Autodesk Inventor part; units mm, degrees
ref_plane "YZ Plane" through (0, 0, 0) normal (1, 0, 0) x (0, 1, 0)
ref_plane "XZ Plane" through (0, 0, 0) normal (0, 1, 0) x (-1, 0, 0)
ref_plane "XY Plane" through (0, 0, 0) normal (0, 0, 1) x (1, 0, 0)
sketch "Sketch1" plane through (0, 0, 0) normal (0, 1, 0) x (-1, 0, 0)
  line L0 (-600, 400) -> (600, 400)
  line L1 (600, 400) -> (600, -400)
  line L2 (600, -400) -> (-600, -400)
  line L3 (-600, -400) -> (-600, 400)
  line L4 (-600, 400) -> (600, -400) construction
  line L5 (600, 400) -> (-600, -400) construction
  point P0 (0, 0)
  dimension "d0" = 1200
  dimension "d1" = 800
extrude "Extrusion1" add sketch "Sketch1" along normal blind 35
sketch "Sketch2" plane through (0, 35, 0) normal (0, 1, 0) x (1, 0, 0)
  line L0 (-300, -215) -> (300, -215)
  line L1 (300, -215) -> (300, 215)
  line L2 (300, 215) -> (-300, 215)
  line L3 (-300, 215) -> (-300, -215)
  line L4 (-300, -215) -> (300, 215) construction
  line L5 (300, -215) -> (-300, 215) construction
  point P0 (0, 0)
  dimension "d8" = 430
  dimension "d9" = 600
extrude "Extrusion2" cut sketch "Sketch2" against normal blind 35
fillet "Fillet2" radius 10 4 edges at (0, 35, 400) (-600, 35, 0) (0, 35, -400) (600, 35, 0)
fillet "Fillet3" radius 10 8 edges at (597.0711, 32.0711, 397.0711) (600, 12.5, 400) (597.0711, 32.0711, -397.0711) (600, 12.5, -400) (-597.0711, 32.0711, 397.0711) (-600, 12.5, 400) (-597.0711, 32.0711, -397.0711) (-600, 12.5, -400)
properties part number "señales_tapa_x10"
Geometry check sheet. Reference: the model listing, model coordinates, mm. A direction names the side the tool comes from. Round coordinates to 2 decimals unless told otherwise and drop trailing zeros. Order: outer loops, then holes, each group sorted by start corner. A loop starts at its lowest first (then second) coordinate and runs counter-clockwise, first axis right, second up. Notation, with made-up numbers: (-32, -24.5) - (18, -24.5) arc R21 cw to (18, 10.5) - close; hole circle Ø5 at (34.25, -11.5). An arc over 180 degrees is marked (long way). Use a Markdown table: item, result. Add a question column.
1) Thickness scan on line 1 along X through (y, z) = (14.5, -20); line 2 along Z through (x, y) = (-105, 25); line 3 along X through (y, z) = (31.5, 132). Record the ranges inside material, lowest first.
2) Section check A-A (x = 113). Record the cut outline in (y, z), then the cut area to 3 significant figures.
3) Mould release check, pull along Z, two halves, no side actions. Record for faces 3 (the flat face through (8, 12, 400)), 4 (the flat face through (8, 0, 272)), 5 (the flat face through (-300, 18, -3)), 6 (the flat face through (-8, 12, -400)): released by +Z, released by -Z, zero draft, split by the parting line, or undercut.
4) Set-up check for faces 1 (the flat face through (600, 12, -5)), 2 (the flat face through (300, 18, 3)): record each of +Z, -Z, +X, -X, +Y, -Y from which the full face is reachable in a straight line by a thin tool's end or side.
5) Section check C-C (y = 19). Record the cut outline in (x, z).
6) Section check B-B (z = -52). Record the cut outline in (x, y), then the cut area to 3 significant figures.
Established:
| question | item | result |
|---|---|---|
| 1 | line 1 | -600 to -300, 300 to 600 |
| 1 | line 2 | -400 to -215, 215 to 400 |
| 1 | line 3 | -597.6 to -300, 300 to 597.6 |
| 2 | outline | (0, -400) - (25, -400) arc R10 ccw to (35, -390) - (35, -215) - (0, -215) - close; (0, 215) - (35, 215) - (35, 390) arc R10 ccw to (25, 400) - (0, 400) - close |
| 2 | area | 12,900 mm2 |
| 3 | face 3 | released by +Z |
| 3 | face 4 | zero draft |
| 3 | face 5 | undercut |
| 3 | face 6 | released by -Z |
| 4 | face 1 | +Z, -Z, +X, +Y, -Y |
| 4 | face 2 | +Y, -Y |
| 5 | outline | (-600, -390) arc R10 ccw to (-590, -400) - (590, -400) arc R10 ccw to (600, -390) - (600, 390) arc R10 ccw to (590, 400) - (-590, 400) arc R10 ccw to (-600, 390) - close; hole (-300, -215) - (300, -215) - (300, 215) - (-300, 215) - close |
| 6 | outline | (-600, 0) - (-300, 0) - (-300, 35) - (-590, 35) arc R10 ccw to (-600, 25) - close; (300, 0) - (600, 0) - (600, 25) arc R10 ccw to (590, 35) - (300, 35) - close |
| 6 | area | 21,000 mm2 |
